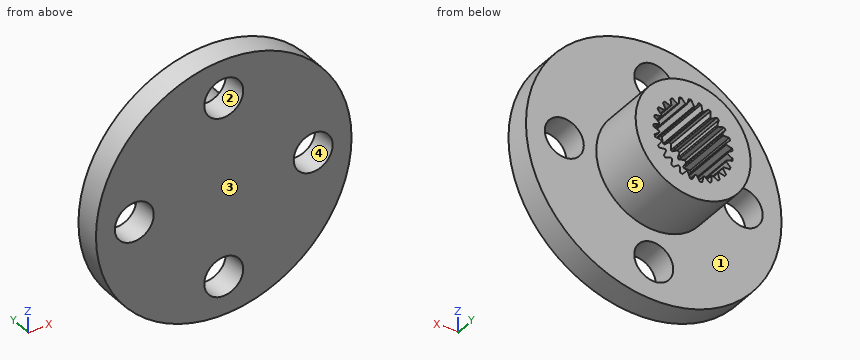
from build123d import *

# Parameters (mm, degrees)
SKETCH1_R           = 4.5
BOSS_EXTRUDE1_DEPTH = 6.5
SKETCH2_R           = 10
BOSS_EXTRUDE2_DEPTH = 2
SKETCH3_R           = 1.525
CUT_EXTRUDE1_DEPTH  = 7.5


with BuildPart() as part:
    # Sketch1 → Boss-Extrude1 (new body)
    with BuildSketch(Plane(origin=(24.301487189, 0, -59.250523978), x_dir=(0.955627849, 0, 0.29457667), z_dir=(0, -1, 0))):
        Circle(SKETCH1_R)
        with BuildLine():
            Line((-1.743463309, 2.563266606), (-1.337804671, 2.314678673))
            ThreePointArc((-1.337804671, 2.314678673), (-1.287955514, 2.342782383), (-1.237516253, 2.369812698))
            Line((-1.237516253, 2.369812698), (-1.230043219, 2.845521688))
            ThreePointArc((-1.230043219, 2.845521688), (-1.141186113, 2.882307106), (-1.05123072, 2.916318565))
            Line((-1.05123072, 2.916318565), (-0.7201379, 2.574657279))
            ThreePointArc((-0.7201379, 2.574657279), (-0.664865737, 2.589481077), (-0.609288952, 2.603118451))
            Line((-0.609288952, 2.603118451), (-0.483746682, 3.062023701))
            ThreePointArc((-0.483746682, 3.062023701), (-0.388533024, 3.075555574), (-0.292945439, 3.086127504))
            Line((-0.292945439, 3.086127504), (-0.057222215, 2.672860699))
            ThreePointArc((-0.057222215, 2.672860699), (0, 2.673473153), (0.057222215, 2.672860699))
            Line((0.057222215, 2.672860699), (0.292945439, 3.086127504))
            ThreePointArc((0.292945439, 3.086127504), (0.388533024, 3.075555574), (0.483746682, 3.062023701))
            Line((0.483746682, 3.062023701), (0.609288952, 2.603118451))
            ThreePointArc((0.609288952, 2.603118451), (0.664865737, 2.589481077), (0.7201379, 2.574657279))
            Line((0.7201379, 2.574657279), (1.05123072, 2.916318565))
            ThreePointArc((1.05123072, 2.916318565), (1.141186113, 2.882307106), (1.230043219, 2.845521688))
            Line((1.230043219, 2.845521688), (1.237516253, 2.369812698))
            ThreePointArc((1.237516253, 2.369812698), (1.287955514, 2.342782383), (1.337804671, 2.314678673))
            Line((1.337804671, 2.314678673), (1.743463309, 2.563266606))
            ThreePointArc((1.743463309, 2.563266606), (1.822134282, 2.507952683), (1.899051617, 2.450225083))
            Line((1.899051617, 2.450225083), (1.787985857, 1.987602897))
            ThreePointArc((1.787985857, 1.987602897), (1.830118309, 1.948878055), (1.871412256, 1.909260293))
            Line((1.871412256, 1.909260293), (2.326147686, 2.049155178))
            ThreePointArc((2.326147686, 2.049155178), (2.388591053, 1.976014368), (2.448735618, 1.900971824))
            Line((2.448735618, 1.900971824), (2.226109733, 1.480504696))
            ThreePointArc((2.226109733, 1.480504696), (2.257288041, 1.432518551), (2.287432125, 1.383876068))
            Line((2.287432125, 1.383876068), (2.762671649, 1.406287795))
            ThreePointArc((2.762671649, 1.406287795), (2.804963863, 1.319915804), (2.844556554, 1.232273514))
            Line((2.844556554, 1.232273514), (2.524358948, 0.88038094))
            ThreePointArc((2.524358948, 0.88038094), (2.542624063, 0.826148638), (2.559724222, 0.771537819))
            Line((2.559724222, 0.771537819), (3.025606792, 0.675058177))
            ThreePointArc((3.025606792, 0.675058177), (3.045090477, 0.580882075), (3.06164354, 0.486146927))
            Line((3.06164354, 0.486146927), (2.663993406, 0.224939612))
            ThreePointArc((2.663993406, 0.224939612), (2.668197664, 0.167868768), (2.671179432, 0.110721012))
            Line((2.671179432, 0.110721012), (3.098431932, -0.098587829))
            ThreePointArc((3.098431932, -0.098587829), (3.093882858, -0.194650611), (3.086356203, -0.290526059))
            Line((3.086356203, -0.290526059), (2.636239362, -0.444635499))
            ThreePointArc((2.636239362, -0.444635499), (2.626118593, -0.500958914), (2.614794614, -0.557052804))
            Line((2.614794614, -0.557052804), (2.9765712, -0.866039198))
            ThreePointArc((2.9765712, -0.866039198), (2.948275201, -0.957952683), (2.917141754, -1.048944224))
            Line((2.917141754, -1.048944224), (2.442840702, -1.086272527))
            ThreePointArc((2.442840702, -1.086272527), (2.419030833, -1.138309505), (2.394112634, -1.189824943))
            Line((2.394112634, -1.189824943), (2.667681551, -1.57907414))
            ThreePointArc((2.667681551, -1.57907414), (2.617416569, -1.661063064), (2.564632561, -1.741453366))
            Line((2.564632561, -1.741453366), (2.095949377, -1.659655056))
            ThreePointArc((2.095949377, -1.659655056), (2.059946468, -1.704135923), (2.022999752, -1.747836005))
            Line((2.022999752, -1.747836005), (2.19117166, -2.192890046))
            ThreePointArc((2.19117166, -2.192890046), (2.122096028, -2.259802745), (2.050978072, -2.324540589))
            Line((2.050978072, -2.324540589), (1.617361845, -2.128755355))
            ThreePointArc((1.617361845, -2.128755355), (1.571428092, -2.162885215), (1.524774356, -2.196024103))
            Line((1.524774356, -2.196024103), (1.576982395, -2.668918606))
            ThreePointArc((1.576982395, -2.668918606), (1.49343639, -2.716550708), (1.408453087, -2.761568377))
            Line((1.408453087, -2.761568377), (1.037149519, -2.464098126))
            ThreePointArc((1.037149519, -2.464098126), (0.984171108, -2.485732473), (0.930741779, -2.50622793))
            Line((0.930741779, -2.50622793), (0.863705526, -2.977249194))
            ThreePointArc((0.863705526, -2.977249194), (0.77093865, -3.002607799), (0.677429816, -3.025076668))
            Line((0.677429816, -3.025076668), (0.391769275, -2.644612549))
            ThreePointArc((0.391769275, -2.644612549), (0.335075035, -2.652392018), (0.278227274, -2.658956239))
            Line((0.278227274, -2.658956239), (0.096158863, -3.098508266))
            ThreePointArc((0.096158863, -3.098508266), (0, -3.1), (-0.096158863, -3.098508266))
            Line((-0.096158863, -3.098508266), (-0.278227274, -2.658956239))
            ThreePointArc((-0.278227274, -2.658956239), (-0.335075035, -2.652392018), (-0.391769275, -2.644612549))
            Line((-0.391769275, -2.644612549), (-0.677429816, -3.025076668))
            ThreePointArc((-0.677429816, -3.025076668), (-0.77093865, -3.002607799), (-0.863705526, -2.977249194))
            Line((-0.863705526, -2.977249194), (-0.930741779, -2.50622793))
            ThreePointArc((-0.930741779, -2.50622793), (-0.984171108, -2.485732473), (-1.037149519, -2.464098126))
            Line((-1.037149519, -2.464098126), (-1.408453087, -2.761568377))
            ThreePointArc((-1.408453087, -2.761568377), (-1.49343639, -2.716550708), (-1.576982395, -2.668918606))
            Line((-1.576982395, -2.668918606), (-1.524774356, -2.196024103))
            ThreePointArc((-1.524774356, -2.196024103), (-1.571428092, -2.162885215), (-1.617361845, -2.128755355))
            Line((-1.617361845, -2.128755355), (-2.050978072, -2.324540589))
            ThreePointArc((-2.050978072, -2.324540589), (-2.122096028, -2.259802745), (-2.19117166, -2.192890046))
            Line((-2.19117166, -2.192890046), (-2.022999752, -1.747836005))
            ThreePointArc((-2.022999752, -1.747836005), (-2.059946468, -1.704135923), (-2.095949377, -1.659655056))
            Line((-2.095949377, -1.659655056), (-2.564632561, -1.741453366))
            ThreePointArc((-2.564632561, -1.741453366), (-2.617416569, -1.661063064), (-2.667681551, -1.57907414))
            Line((-2.667681551, -1.57907414), (-2.394112634, -1.189824943))
            ThreePointArc((-2.394112634, -1.189824943), (-2.419030833, -1.138309505), (-2.442840702, -1.086272527))
            Line((-2.442840702, -1.086272527), (-2.917141754, -1.048944224))
            ThreePointArc((-2.917141754, -1.048944224), (-2.948275201, -0.957952683), (-2.9765712, -0.866039198))
            Line((-2.9765712, -0.866039198), (-2.614794614, -0.557052804))
            ThreePointArc((-2.614794614, -0.557052804), (-2.626118593, -0.500958914), (-2.636239362, -0.444635499))
            Line((-2.636239362, -0.444635499), (-3.086356203, -0.290526059))
            ThreePointArc((-3.086356203, -0.290526059), (-3.093882858, -0.194650611), (-3.098431932, -0.098587829))
            Line((-3.098431932, -0.098587829), (-2.671179432, 0.110721012))
            ThreePointArc((-2.671179432, 0.110721012), (-2.668197664, 0.167868768), (-2.663993406, 0.224939612))
            Line((-2.663993406, 0.224939612), (-3.06164354, 0.486146927))
            ThreePointArc((-3.06164354, 0.486146927), (-3.045090477, 0.580882075), (-3.025606792, 0.675058177))
            Line((-3.025606792, 0.675058177), (-2.559724222, 0.771537819))
            ThreePointArc((-2.559724222, 0.771537819), (-2.542624063, 0.826148638), (-2.524358948, 0.88038094))
            Line((-2.524358948, 0.88038094), (-2.844556554, 1.232273514))
            ThreePointArc((-2.844556554, 1.232273514), (-2.804963863, 1.319915804), (-2.762671649, 1.406287795))
            Line((-2.762671649, 1.406287795), (-2.287432125, 1.383876068))
            ThreePointArc((-2.287432125, 1.383876068), (-2.257288041, 1.432518551), (-2.226109733, 1.480504696))
            Line((-2.226109733, 1.480504696), (-2.448735618, 1.900971824))
            ThreePointArc((-2.448735618, 1.900971824), (-2.388591053, 1.976014368), (-2.326147686, 2.049155178))
            Line((-2.326147686, 2.049155178), (-1.871412256, 1.909260293))
            ThreePointArc((-1.871412256, 1.909260293), (-1.830118309, 1.948878055), (-1.787985857, 1.987602897))
            Line((-1.787985857, 1.987602897), (-1.899051617, 2.450225083))
            ThreePointArc((-1.899051617, 2.450225083), (-1.822134282, 2.507952683), (-1.743463309, 2.563266606))
        make_face(mode=Mode.SUBTRACT)
    extrude(amount=-BOSS_EXTRUDE1_DEPTH)

    # Sketch2 → Boss-Extrude2 (add)
    with BuildSketch(Plane(origin=(0, 0, 0), x_dir=(-1, 0, 0), z_dir=(0, -1, 0))):
        with Locations((-24.301487189, 59.250523978)):
            Circle(SKETCH2_R)
    extrude(amount=-BOSS_EXTRUDE2_DEPTH)

    # Sketch3 → Cut-Extrude1 (cut, through all)
    with BuildSketch(Plane(origin=(0, 0, 0), x_dir=(-1, 0, 0), z_dir=(0, -1, 0))):
        with Locations((-24.301487189, 66.250523978)):
            Circle(SKETCH3_R)
        with Locations((-17.301487189, 59.250523978)):
            Circle(SKETCH3_R)
        with Locations((-24.301487189, 52.250523978)):
            Circle(SKETCH3_R)
        with Locations((-31.301487189, 59.250523978)):
            Circle(SKETCH3_R)
    extrude(amount=-CUT_EXTRUDE1_DEPTH, mode=Mode.SUBTRACT)


solid = part.part
CAD build for the part. Positions are in the model's coordinates, mm. Face numbers are marked on the shaded views. A direction names the side the tool comes from. Round coordinates to 2 decimals unless told otherwise and drop trailing zeros. Loops run counter-clockwise (first coordinate to the right, second up) from the corner with the lowest first, then second, coordinate; pieces in that order, holes last. Notation, with made-up numbers: M 82,-36.5 L 116,-36.5 A29 cw 116,-14.5 Z; hole C 57.5,84 d3. An arc over 180 degrees is marked long. One line per question, with ' | ' between items. Start each with the question number.
Item 1: Pin check, flat tips, straight feed: pin 1 Ø3 at (x, z) = (25, -59.5) entering from +Y; pin 2 Ø2.5 at (x, z) = (17.3, -59.25) entering from -Y; pin 3 Ø10 at (x, z) = (32, -60.5) entering from +Y; pin 4 Ø1.5 at (y, z) = (1, -52.5) entering from -X. Stop position of each tip, or through.
Item 2: Cut at A-A, the plane z = -52. Write the cut outline in (x, y), plus the area to 3 significant figures.
Item 3: Two-plate mould, pull along Z, no slides. Class the marked faces 3, 4 and 5: pulls with the +Z half, pulls with the -Z half, needs draft (parallel to the pull), parting line crosses it, or undercut.
Item 4: Which spindle directions (+Z, -Z, +X, -X, +Y, -Y) get a long thin tool onto all of the face, cutting with end or side? Do the marked faces 1 and 2. Say none if no direction does.
Item 5: Wall check: line 1 (Y direction, x = 21.75, z = -66.25); line 2 (Z direction, x = 31.25, y = 1.75); line 3 (Z direction, x = 16.5, y = 1.25). Give the ranges that are in metal, low to high.
Item 6: Cut at C-C, the plane z = -55.5. Write the cut outline in (x, y), plus the area to 3 significant figures.
Item 7: Cut at B-B, the plane x = 17.25. Write the cut outline in (y, z), plus the area to 3 significant figures.
Responses:
1) pin 1: stops at y = 2 | pin 2: passes through | pin 3: stops at y = 6.5 | pin 4: stops at x = 16.3
2) outline: M 17.41,0 L 22.8,0 L 22.8,2 L 17.41,2 Z; M 25.81,0 L 31.19,0 L 31.19,2 L 25.81,2 Z | area: 21.5 mm²
3) face 3: needs draft | face 4: undercut | face 5: parting line crosses it
4) face 1: +Y | face 2: +Y, -Y
5) line 1: y = 0 to 2 | line 2: z = -66.44 to -60.77, -57.73 to -52.06 | line 3: z = -65.51 to -60.55, -57.95 to -52.99
6) outline: M 15.03,0 L 33.57,0 L 33.57,2 L 26.79,2 L 26.79,6.5 L 21.81,6.5 L 21.81,2 L 15.03,2 Z | area: 59.5 mm²
7) outline: M 0,-66.34 L 2,-66.34 L 2,-60.77 L 0,-60.77 Z; M 0,-57.73 L 2,-57.73 L 2,-52.16 L 0,-52.16 Z | area: 22.3 mm²
